Could you check a few things on this model? Use its own coordinates, in mm. A direction names the side the tool comes from. Give positions to 0.01 mm unless a question says otherwise; leave off trailing zeros. Order: outer loops, then holes, each group sorted by start corner. A loop starts at its lowest first (then second) coordinate and runs counter-clockwise, first axis right, second up. Notation, with made-up numbers: (-34.5, 84) -> (-18.5, 84) arc R16 ccw to (-18.5, 106) -> close; hole circle Ø6 at (40.25, -10.75). An arc over 180 degrees is marked (long way). Write each question's results on one line, items separated by ' | '.
```python
from build123d import *

# Parameters (mm, degrees)
SKETCH1_R            = 6
SKETCH1_R_2          = 1.45
BOSS_EXTRUDE1_DEPTH  = 3
SKETCH2_R            = 20
SKETCH2_R_2          = 1.45
BOSS_EXTRUDE2_DEPTH  = 2
SKETCH3_R            = 12
SKETCH3_R_2          = 6
BOSS_EXTRUDE3_DEPTH  = 2
BOSS_EXTRUDE4_DEPTH  = 11
SKETCH5_R            = 4
SKETCH5_R_2          = 1.3
BOSS_EXTRUDE5_DEPTH  = 9
SKETCH6_R            = 4
SKETCH6_R_2          = 1.3
BOSS_EXTRUDE6_DEPTH  = 9
SKETCH7_R            = 4
SKETCH7_R_2          = 1.3
BOSS_EXTRUDE7_DEPTH  = 9
SKETCH8_R            = 4.5
SKETCH8_R_2          = 1.3
BOSS_EXTRUDE8_DEPTH  = 14
SKETCH9_R            = 4.5
SKETCH9_R_2          = 1.3
BOSS_EXTRUDE9_DEPTH  = 14
SKETCH10_R           = 4.5
SKETCH10_R_2         = 1.3
BOSS_EXTRUDE10_DEPTH = 14
SKETCH11_R           = 4.5
SKETCH11_R_2         = 1.3
BOSS_EXTRUDE11_DEPTH = 14
SKETCH12_R           = 7.6
CUT_EXTRUDE1_DEPTH   = 5
SKETCH13_R           = 8.05
CUT_EXTRUDE2_DEPTH   = 4.5


with BuildPart() as part:
    # Sketch1 → Boss-Extrude1 (new body)
    with BuildSketch(Plane.XY.offset(344.5)):
        with BuildLine():
            Line((277.006534343, 300.548212638), (273.908821488, 170.622068635))
            ThreePointArc((273.908821488, 170.622068635), (300, 143.901406829), (326.091178512, 170.622068635))
            Line((326.091178512, 170.622068635), (322.993465657, 300.548212638))
            ThreePointArc((322.993465657, 300.548212638), (300, 323), (277.006534343, 300.548212638))
        make_face()
        with Locations((300, 170)):
            Circle(SKETCH1_R, mode=Mode.SUBTRACT)
        with Locations((300, 313.5)):
            Circle(SKETCH1_R_2, mode=Mode.SUBTRACT)
        with Locations((288.308657049, 293.25)):
            Circle(SKETCH1_R_2, mode=Mode.SUBTRACT)
        with Locations((311.691342951, 293.25)):
            Circle(SKETCH1_R_2, mode=Mode.SUBTRACT)
        with BuildLine():
            Line((305, 258.3), (314, 258.3))
            ThreePointArc((314, 258.3), (315.7, 260), (314, 261.7))
            Line((314, 261.7), (305, 261.7))
            ThreePointArc((305, 261.7), (303.3, 260), (305, 258.3))
        make_face(mode=Mode.SUBTRACT)
        with BuildLine():
            Line((294.661250685, 252.292425307), (293.257422469, 237.959091974))
            ThreePointArc((293.257422469, 237.959091974), (294.02083171, 235.651384543), (296.243136361, 234.666666667))
            Line((296.243136361, 234.666666667), (303.756863639, 234.666666667))
            ThreePointArc((303.756863639, 234.666666667), (305.97916829, 235.651384543), (306.742577531, 237.959091974))
            Line((306.742577531, 237.959091974), (305.338749315, 252.292425307))
            ThreePointArc((305.338749315, 252.292425307), (304.368317547, 254.222304651), (302.353035423, 255))
            Line((302.353035423, 255), (297.646964577, 255))
            ThreePointArc((297.646964577, 255), (295.631682453, 254.222304651), (294.661250685, 252.292425307))
        make_face(mode=Mode.SUBTRACT)
        with BuildLine():
            Line((292.180065932, 226.959091974), (290.776237716, 212.625758641))
            ThreePointArc((290.776237716, 212.625758641), (291.539646956, 210.318051209), (293.761951607, 209.333333333))
            Line((293.761951607, 209.333333333), (306.238048393, 209.333333333))
            ThreePointArc((306.238048393, 209.333333333), (308.460353044, 210.318051209), (309.223762284, 212.625758641))
            Line((309.223762284, 212.625758641), (307.819934068, 226.959091974))
            ThreePointArc((307.819934068, 226.959091974), (306.849502301, 228.888971317), (304.834220177, 229.666666667))
            Line((304.834220177, 229.666666667), (295.165779823, 229.666666667))
            ThreePointArc((295.165779823, 229.666666667), (293.150497699, 228.888971317), (292.180065932, 226.959091974))
        make_face(mode=Mode.SUBTRACT)
        with BuildLine():
            Line((289.698881178, 201.625758641), (288.295052962, 187.292425307))
            ThreePointArc((288.295052962, 187.292425307), (289.058462202, 184.984717876), (291.280766853, 184))
            Line((291.280766853, 184), (308.719233147, 184))
            ThreePointArc((308.719233147, 184), (310.941537798, 184.984717876), (311.704947038, 187.292425307))
            Line((311.704947038, 187.292425307), (310.301118822, 201.625758641))
            ThreePointArc((310.301118822, 201.625758641), (309.330687055, 203.555637984), (307.315404931, 204.333333333))
            Line((307.315404931, 204.333333333), (292.684595069, 204.333333333))
            ThreePointArc((292.684595069, 204.333333333), (290.669312945, 203.555637984), (289.698881178, 201.625758641))
        make_face(mode=Mode.SUBTRACT)
    extrude(amount=BOSS_EXTRUDE1_DEPTH)

    # Sketch2 → Boss-Extrude2 (add)
    with BuildSketch(Plane.XY.offset(342.5)):
        with Locations((300, 300)):
            Circle(SKETCH2_R)
        with Locations((300, 313.5)):
            Circle(SKETCH2_R_2, mode=Mode.SUBTRACT)
        with Locations((288.308657049, 293.25)):
            Circle(SKETCH2_R_2, mode=Mode.SUBTRACT)
        with Locations((311.691342951, 293.25)):
            Circle(SKETCH2_R_2, mode=Mode.SUBTRACT)
    extrude(amount=BOSS_EXTRUDE2_DEPTH)

    # Sketch3 → Boss-Extrude3 (add)
    with BuildSketch(Plane.XY.offset(342.5)):
        with Locations((300, 170)):
            Circle(SKETCH3_R)
        with Locations((300, 170)):
            Circle(SKETCH3_R_2, mode=Mode.SUBTRACT)
    extrude(amount=BOSS_EXTRUDE3_DEPTH)

    # Sketch4 → Boss-Extrude4 (add)
    with BuildSketch(Plane.XY.offset(333.5)):
        with BuildLine():
            Line((277.006534343, 300.548212638), (273.908821488, 170.622068635))
            ThreePointArc((273.908821488, 170.622068635), (300, 143.901406829), (326.091178512, 170.622068635))
            Line((326.091178512, 170.622068635), (322.993465657, 300.548212638))
            ThreePointArc((322.993465657, 300.548212638), (300, 323), (277.006534343, 300.548212638))
        make_face()
        with BuildLine():
            Line((282.510952348, 300.619041388), (277.9152372, 170.781711074))
            ThreePointArc((277.9152372, 170.781711074), (300, 147.901406829), (322.0847628, 170.781711074))
            Line((322.0847628, 170.781711074), (317.489047652, 300.619041388))
            ThreePointArc((317.489047652, 300.619041388), (300, 317.5), (282.510952348, 300.619041388))
        make_face(mode=Mode.SUBTRACT)
    extrude(amount=BOSS_EXTRUDE4_DEPTH)

    # Sketch5 → Boss-Extrude5 (add)
    with BuildSketch(Plane.XY.offset(333.5)):
        with Locations((312.124355653, 307)):
            Circle(SKETCH5_R)
        with Locations((312.124355653, 307)):
            Circle(SKETCH5_R_2, mode=Mode.SUBTRACT)
    extrude(amount=BOSS_EXTRUDE5_DEPTH)

    # Sketch6 → Boss-Extrude6 (add)
    with BuildSketch(Plane.XY.offset(333.5)):
        with Locations((287.875644347, 307)):
            Circle(SKETCH6_R)
        with Locations((287.875644347, 307)):
            Circle(SKETCH6_R_2, mode=Mode.SUBTRACT)
    extrude(amount=BOSS_EXTRUDE6_DEPTH)

    # Sketch7 → Boss-Extrude7 (add)
    with BuildSketch(Plane.XY.offset(333.5)):
        with Locations((300, 286)):
            Circle(SKETCH7_R)
        with Locations((300, 286)):
            Circle(SKETCH7_R_2, mode=Mode.SUBTRACT)
    extrude(amount=BOSS_EXTRUDE7_DEPTH)

    # Sketch8 → Boss-Extrude8 (add)
    with BuildSketch(Plane.XY.offset(333.5)):
        with Locations((273.593173433, 220)):
            Circle(SKETCH8_R)
        with Locations((273.593173433, 220)):
            Circle(SKETCH8_R_2, mode=Mode.SUBTRACT)
    extrude(amount=BOSS_EXTRUDE8_DEPTH)

    # Sketch9 → Boss-Extrude9 (add)
    with BuildSketch(Plane.XY.offset(333.5)):
        with Locations((326.406826567, 220)):
            Circle(SKETCH9_R)
        with Locations((326.406826567, 220)):
            Circle(SKETCH9_R_2, mode=Mode.SUBTRACT)
    extrude(amount=BOSS_EXTRUDE9_DEPTH)

    # Sketch10 → Boss-Extrude10 (add)
    with BuildSketch(Plane.XY.offset(333.5)):
        with Locations((271.401406829, 170)):
            Circle(SKETCH10_R)
        with Locations((271.401406829, 170)):
            Circle(SKETCH10_R_2, mode=Mode.SUBTRACT)
    extrude(amount=BOSS_EXTRUDE10_DEPTH)

    # Sketch11 → Boss-Extrude11 (add)
    with BuildSketch(Plane.XY.offset(333.5)):
        with Locations((328.598593171, 170)):
            Circle(SKETCH11_R)
        with Locations((328.598593171, 170)):
            Circle(SKETCH11_R_2, mode=Mode.SUBTRACT)
    extrude(amount=BOSS_EXTRUDE11_DEPTH)

    # Sketch12 → Cut-Extrude1 (cut)
    with BuildSketch(Plane.XY.offset(342.5)):
        with Locations((300, 300)):
            Circle(SKETCH12_R)
    extrude(amount=CUT_EXTRUDE1_DEPTH, mode=Mode.SUBTRACT)

    # Sketch13 → Cut-Extrude2 (cut)
    with BuildSketch(Plane.XY.offset(342.5)):
        with Locations((300, 170)):
            Circle(SKETCH13_R)
    extrude(amount=CUT_EXTRUDE2_DEPTH, mode=Mode.SUBTRACT)


solid = part.part
```
Q1. Suppose I cut it at B-B on y = 240.5. Please give me the cut outline in (x, z).
Here are the results:
outline: (275.57, 333.5) -> (280.38, 333.5) -> (280.38, 344.5) -> (293.51, 344.5) -> (293.51, 347.5) -> (275.57, 347.5) -> close; (306.49, 344.5) -> (319.62, 344.5) -> (319.62, 333.5) -> (324.43, 333.5) -> (324.43, 347.5) -> (306.49, 347.5) -> close
Q2. Suppose I cut it at A-A on z = 337.25. State how many separate pieces and enclosed holes the cut face has, and give its area (3 significant figures).
Here are the results:
separate pieces: 2 | enclosed holes: 8 | area: 2,190 mm²
Q3. For faces 1 (the flat face through (310, 220, 344.5)), 2 (the cylindrical face through (304.39, 254.2, 345.98)), which set-ups out of +Z, -Z, +X, -X, +Y, -Y let a thin tool reach every point of the face, with its end or its side?
Here are the results:
face 1: -Z | face 2: +Z, -Z
Q4. Thinking about a two-plate mould opening in Y: for faces 3 (the cylindrical face through (291.156, 178.11, 343.486)), 4 (the cylindrical face through (300, 323, 340)), 5 (the cylindrical face through (289.035, 185.011, 345.979)), which applies, +Y half, -Y half, draft (parallel to the pull), parting line (faces both ways), or undercut?
Here are the results:
face 3: undercut | face 4: +Y half | face 5: undercut
Q5. Suppose I cut it at C-C on y = 278. Please give me the cut outline in (x, z), and give its area (3 significant figures).
Here are the results:
outline: (276.47, 333.5) -> (281.71, 333.5) -> (281.71, 344.5) -> (318.29, 344.5) -> (318.29, 333.5) -> (323.53, 333.5) -> (323.53, 347.5) -> (276.47, 347.5) -> close | area: 256 mm²
Q6. I need wall thicknesses on line 1 along X through (y, z) = (300, 345.8); line 2 along Y through (x, z) = (300, 340.75); line 3 along Y through (x, z) = (299.5, 341). Which ranges of each line are inside material? Lowest first, please.
Here are the results:
line 1: x = 276.99 to 292.4, 307.6 to 323.01 | line 2: y = 143.9 to 147.9, 282 to 284.7, 287.3 to 290, 317.5 to 323 | line 3: y = 143.91 to 147.91, 282.03 to 284.8, 287.2 to 289.97, 317.49 to 322.99
Q7. I'm going to push flat-ended pins straight in: pin 1 Ø0.9 at (x, z) = (296.5, 346.5) entering from +Y; pin 2 Ø4 at (x, z) = (291.5, 341.5) entering from -Y; pin 3 Ø8 at (x, y) = (302.5, 170.5) entering from -Z. Where does each tip first touch, or does it pass through?
Here are the results:
pin 1: stops at y = 322.8 | pin 2: stops at y = 144.72 | pin 3: stops at z = 347
